Work out the finished part from the listing and answer in its coordinate system (mm). A direction names the side the tool comes from. Coordinates: 2 decimals unless noted, no trailing zeros. Order: outer loops, then holes, each group sorted by start corner. A loop starts at its lowest first (then second) coordinate and runs counter-clockwise, first axis right, second up.
```python
from build123d import *

# Parameters (mm, degrees)
F0_R      = 5.3136453871
F1_DEPTH  = 12.7
F2_W      = 20.7254816778
F2_H      = 14.2186461017
F2_H_2    = 13.4956622496
F3_DEPTH  = 50.8
F4_R      = 5.08
F5_R      = 4.4744147094
F6_DEPTH  = 25.4
F7_R      = 4.4306212016
F8_DEPTH  = 25.4
F9_W      = 20.7254816778
F9_H      = 10.515610534
F10_DEPTH = 25.4
F12_DEPTH = 25.4


with BuildPart() as f1:
    # F0 (on Front) → F1 (new body)
    with BuildSketch(Plane.XZ):
        with BuildLine():
            ThreePointArc((10.7242334634, 39.4025146961), (-6.1453450471, 54.1304557314), (-23.0149235576, 39.4025146961))
            Line((-23.0149235576, 39.4025146961), (-23.0149235576, -36.0286012292))
            ThreePointArc((-23.0149235576, -36.0286012292), (-6.1453450471, -50.7565422645), (10.7242334634, -36.0286012292))
            Line((10.7242334634, -36.0286012292), (10.7242334634, 39.4025146961))
        make_face()
        with Locations((-6.1453450471, -33.7312525427)):
            Circle(F0_R, mode=Mode.SUBTRACT)
        with Locations((-6.1453450471, 37.1051660096)):
            Circle(F0_R, mode=Mode.SUBTRACT)
    extrude(amount=F1_DEPTH)

    # F2 (on Front) → F3 (join)
    with BuildSketch(Plane.XZ):
        with Locations((-5.9043520596, 18.5565375723)):
            Rectangle(F2_W, F2_H)
        with Locations((-5.9043520596, -16.0261015408)):
            Rectangle(F2_W, F2_H_2)
    extrude(amount=F3_DEPTH)

    # F4
    f4_edges = [f1.edges().sort_by_distance(p)[0] for p in [
        (4.458389, -50.8, 18.556538),
        (-16.267093, -50.8, 18.556538),
        (4.458389, -50.8, -16.026102),
        (-16.267093, -50.8, -16.026102),
    ]]
    fillet(f4_edges, radius=F4_R)

    # F5 (on face) → F6 (cut)
    with BuildSketch(Plane(origin=(0, 0, -22.7739326656), x_dir=(1, 0, 0), z_dir=(0, 0, -1))):
        with Locations((-5.9043520596, 41.6847616434)):
            Circle(F5_R)
    extrude(amount=-F6_DEPTH, mode=Mode.SUBTRACT)

    # F7 (on face) → F8 (cut)
    with BuildSketch(Plane(origin=(0, 0, 11.4472145215), x_dir=(1, 0, 0), z_dir=(0, 0, -1))):
        with Locations((-5.9701367281, 41.9478155673)):
            Circle(F7_R)
    extrude(amount=-F8_DEPTH, mode=Mode.SUBTRACT)

    # F9 (on face) → F10 (join)
    with BuildSketch(Plane.XY.offset(-9.278270416)):
        with Locations((-5.9043520596, -17.957805267)):
            Rectangle(F9_W, F9_H)
    extrude(amount=F10_DEPTH)

    # F11 (on face) → F12 (cut)
    with BuildSketch(Plane(origin=(-16.2670928985, 0, 0), x_dir=(0, -1, 0), z_dir=(-1, 0, 0))):
        with BuildLine():
            Line((23.215610534, -9.278270416), (23.215610534, 11.4472145215))
            ThreePointArc((23.215610534, 11.4472145215), (14.6873741611, 1.0844720528), (23.215610534, -9.278270416))
        make_face()
    extrude(amount=-F12_DEPTH, mode=Mode.SUBTRACT)


solid = f1.part
```
1. The part is cut by section C-C (z = -20). Determine the outline of the cut face in (x, y).
2. The part is cut by section D-D (x = -8). Determine the outline of the cut face in (y, z).
3. Flat-ended cylindrical pins translate along their axes: pin 1 (4 mm diameter, centred on x = 3.5, y = -26, fed in from -Z); pin 2 (10.5 mm diameter, centred on x = -7.5, y = -31.5, fed in from +Z); pin 3 (3 mm diameter, centred on x = -16, y = -9, fed in from +Z). Find the tip coordinate at first contact, or state that the pin passes through.
4. The mould has two halves that part along Z. Classify faces 1 (the cylindrical face through (-6.487, -6.261, -50.753)), 2 (the flat face through (-6, -37, -9.278)), 3 (the cylindrical face through (-14.82, -49.27, -15.93)): released by +Z, released by -Z, zero draft, split by the parting line, or undercut.
5. The part is cut by section A-A (y = -39.5). Determine the outline of the cut face in (x, z), plus the area to 3 significant figures.
6. The part is cut by section B-B (x = -3). Determine the outline of the cut face in (y, z), plus the area to 3 significant figures.
7. Consider probe 1 along Z at (x, y) = (-5.5, -28); probe 2 along Y at (x, z) = (4, -28); probe 3 along X at (y, z) = (-9.5, 37). Determine where each line is inside the solid, lowest interval first.
8. For faces 4 (the cylindrical face through (-1.877, -40.251, 18.457)), 5 (the flat face through (-6, -31, 25.666)), 6 (the flat face through (-6, -31, -22.774)), determine the directions among +Z, -Z, +X, -X, +Y, -Y from which every point of the face is accessible in a straight line to the end or side of a thin tool.
Worked out:
1. outline: (-23.01, -12.7) - (-16.27, -12.7) - (-16.27, -45.72) arc R5.08 ccw to (-11.19, -50.8) - (-0.62, -50.8) arc R5.08 ccw to (4.46, -45.72) - (4.46, -12.7) - (10.72, -12.7) - (10.72, 0) - (-23.01, 0) - close; hole circle Ø8.95 at (-5.9, -41.68)
2. outline: (-50.8, -22.77) - (-45.64, -22.77) - (-45.64, -9.28) - (-50.8, -9.28) - close; (-50.8, 11.45) - (-45.89, 11.45) - (-45.89, 25.67) - (-50.8, 25.67) - close; (-38.01, 11.45) - (-23.22, 11.45) arc R10.56 cw to (-23.22, -9.28) - (-37.73, -9.28) - (-37.73, -22.77) - (-12.7, -22.77) - (-12.7, -28.75) - (0, -28.75) - (0, 32.13) - (-12.7, 32.13) - (-12.7, 25.67) - (-38.01, 25.67) - close; (-12.7, -50.66) - (0, -50.66) - (0, -38.71) - (-12.7, -38.71) - close; (-12.7, 42.08) - (0, 42.08) - (0, 54.03) - (-12.7, 54.03) - close
3. pin 1: stops at z = -22.77
3. pin 2: stops at z = 25.67
3. pin 3: stops at z = 51.94
4. face 1: released by -Z
4. face 2: undercut
4. face 3: zero draft
5. outline: (-16.27, -22.77) - (-9.81, -22.77) - (-9.81, -9.28) - (-16.27, -9.28) - close; (-16.27, 11.45) - (-9.66, 11.45) - (-9.66, 25.67) - (-16.27, 25.67) - close; (-2.28, 11.45) - (4.46, 11.45) - (4.46, 25.67) - (-2.28, 25.67) - close; (-2, -22.77) - (4.46, -22.77) - (4.46, -9.28) - (-2, -9.28) - close
5. area: 364 mm2
6. outline: (-50.8, -22.77) - (-45.09, -22.77) - (-45.09, -9.28) - (-50.8, -9.28) - close; (-50.8, 11.45) - (-45.24, 11.45) - (-45.24, 25.67) - (-50.8, 25.67) - close; (-38.66, 11.45) - (-23.22, 11.45) arc R10.56 cw to (-23.22, -9.28) - (-38.28, -9.28) - (-38.28, -22.77) - (-12.7, -22.77) - (-12.7, -29.45) - (0, -29.45) - (0, 32.82) - (-12.7, 32.82) - (-12.7, 25.67) - (-38.66, 25.67) - close; (-12.7, -50.46) - (0, -50.46) - (0, -38.01) - (-12.7, -38.01) - close; (-12.7, 41.39) - (0, 41.39) - (0, 53.84) - (-12.7, 53.84) - close
6. area: 2,060 mm2
7. probe 1: z = -22.77 to -9.28, 11.45 to 25.67
7. probe 2: y = -12.7 to 0
7. probe 3: x = -23.01 to -11.46, -0.83 to 10.72
8. face 4: +Z
8. face 5: +Z, +X, -X, -Y
8. face 6: -Z, +X, -X, -Y
